from build123d import *

# Parameters (mm, degrees)
BOSS_EXTRUDE1_DEPTH = 12.7
CIRPATTERN1_COUNT   = 5
SKETCH3_R           = 3.81
CUT_EXTRUDE1_DEPTH  = 16.42998846


with BuildPart() as part:
    # Sketch1 → Boss-Extrude1 (new body)
    with BuildSketch(Plane(origin=(0, 0, 0), x_dir=(1, 0, 0), z_dir=(0, 1, 0))):
        Polygon((0, 6.35), (6.039208878, 1.962257914), (0, 0), align=None)
    boss_extrude1 = extrude(amount=BOSS_EXTRUDE1_DEPTH)

    # CirPattern1: Boss-Extrude1 ×5 about axis
    cirpattern1_axis = Axis((0, 0, 0), (0, 1, 0))
    for i in range(1, CIRPATTERN1_COUNT):
        add(boss_extrude1.rotate(cirpattern1_axis, i * 360 / CIRPATTERN1_COUNT))

    # Sketch3 → Cut-Extrude1 (cut, through all)
    with BuildSketch(Plane(origin=(0, 12.7, 0), x_dir=(1, 0, 0), z_dir=(0, 1, 0))):
        with Locations(Location((0, 0, 0), (0, 0, 270))):
            Circle(SKETCH3_R)
    extrude(amount=-CUT_EXTRUDE1_DEPTH, mode=Mode.SUBTRACT)


solid = part.part
Input: part model. Units: mm. Frame: model coordinates. Coordinates: 2 decimals unless noted, no trailing zeros. Write each loop counter-clockwise with the first axis right and the second up, starting at its lowest first coordinate (ties: lowest second). Pieces come first, ordered by that corner, then holes. Notation, with made-up numbers: M 69,-12 L 93,-12 A19 ccw 93,9 Z; hole C 32.5,65.25 d6. An arc over 180 degrees is marked long. Answer as a JSON object with one key per item and string values. Group by question number.
(1) Ray query, line 1 along X through (y, z) = (9.5, 0); line 2 along Z through (x, y) = (3, 11.25); line 3 along X through (y, z) = (8, -2). Return the intervals inside material, ascending. Write a range as [from, to].
(2) Section D-D on x = -4.75. Output: boundary loops of the cut face in (y, z), plus the area to 3 significant figures.
(3) Section A-A on y = 10.25. Output: boundary loops of the cut face in (x, z), plus the area to 3 significant figures.
(4) Contact query for flat-ended pins moving along their axis: P1, Ø5, axis at x = -4, y = 10, coming from the -Z side; P2, Ø4, axis at y = 1.5, z = 4, coming from the -X side; P3, Ø6, axis at x = 0, y = 3, coming from the -Z side. Output: stop coordinate, or through.
(5) Section C-C on x = 2.5. Output: boundary loops of the cut face in (y, z).
(6) Mould query, pull axis Z, two halves, no side actions, for faces 1 (the face through (3.778, 6.439, -0.496)), 2 (the face through (2.977, 6.261, -4.187)), 3 (the face through (4.9, 6.26, 1.54)), 4 (the face through (-2, 12.7, -4)). Classes: pulls with the +Z half, pulls with the -Z half, needs draft (parallel to the pull), parting line crosses it, or undercut.
(7) Section B-B on z = -1. Output: boundary loops of the cut face in (x, y), plus the area to 3 significant figures.
Result set:
{
 "1": {"line 1": "x = [-5.4, -3.81], [3.81, 5.4]", "line 2": "z = [-4.17, -2.35], [2.35, 5.14]", "line 3": "x = [-5.99, -3.24], [3.24, 5.99]"},
 "2": {"outline": "M 0,-2.9 L 12.7,-2.9 L 12.7,2.01 L 0,2.01 Z", "area": "62.3 mm2"},
 "3": {"outline": "M -6.04,-1.96 L 0,-6.35 L 6.04,-1.96 L 3.73,5.14 L -3.73,5.14 Z; hole C 0,0 d7.62", "area": "50.3 mm2"},
 "4": {"P1": "stops at z = -5.26", "P2": "stops at x = -4.75", "P3": "stops at z = -6.35"},
 "5": {"outline": "M 0,-4.53 L 12.7,-4.53 L 12.7,-2.88 L 0,-2.88 Z; M 0,2.88 L 12.7,2.88 L 12.7,5.14 L 0,5.14 Z"},
 "6": {"face 1": "undercut", "face 2": "pulls with the -Z half", "face 3": "pulls with the +Z half", "face 4": "needs draft"},
 "7": {"outline": "M -5.73,0 L -3.68,0 L -3.68,12.7 L -5.73,12.7 Z; M 3.68,0 L 5.73,0 L 5.73,12.7 L 3.68,12.7 Z", "area": "52.1 mm2"}
}
